from build123d import *

# Parameters (mm, degrees)
SKETCH_2_R          = 6
SKETCH_2_R_2        = 4
EXTRUDE_1_DEPTH     = 2
SKETCH_4_R          = 25
SKETCH_4_R_2        = 5
SKETCH_4_R_3        = 2
EXTRUDE_3_DEPTH     = 2
SKETCH_3_W          = 24
SKETCH_3_H          = 21.068287801
EXTRUDE_2_DEPTH     = 2
SKETCH_5_R          = 1.5
CUT_EXTRUDE_1_DEPTH = 50.779513859
FILLET_1_R          = 10


with BuildPart() as part:
    # 草图2 → 凸台-拉伸1 (new body)
    with BuildSketch(Plane(origin=(0, 0, 0), x_dir=(1, 0, 0), z_dir=(0, 1, 0))):
        with Locations(Location((0, 0, 0), (0, 0, 270))):
            Circle(SKETCH_2_R)
        with Locations(Location((0, 0, 0), (0, 0, 270))):
            Circle(SKETCH_2_R_2, mode=Mode.SUBTRACT)
    extrude(amount=EXTRUDE_1_DEPTH)

    # 草图4 → 凸台-拉伸3 (add)
    with BuildSketch(Plane(origin=(0, 2, 0), x_dir=(1, 0, 0), z_dir=(0, 1, 0))):
        with Locations(Location((0, 0, 0), (0, 0, 270))):
            Circle(SKETCH_4_R)
        Circle(SKETCH_4_R_2, mode=Mode.SUBTRACT)
        with Locations(Location((-10.253048327, 10.253048327, 0), (0, 0, 270))):
            Circle(SKETCH_4_R_3, mode=Mode.SUBTRACT)
        with Locations(Location((10.253048327, 10.253048327, 0), (0, 0, 270))):
            Circle(SKETCH_4_R_3, mode=Mode.SUBTRACT)
        with Locations(Location((-10.253048327, -10.253048327, 0), (0, 0, 270))):
            Circle(SKETCH_4_R_3, mode=Mode.SUBTRACT)
        with Locations(Location((10.253048327, -10.253048327, 0), (0, 0, 270))):
            Circle(SKETCH_4_R_3, mode=Mode.SUBTRACT)
    extrude(amount=-EXTRUDE_3_DEPTH)

    # 草图3 → 凸台-拉伸2 (add)
    with BuildSketch(Plane(origin=(0, 2, 0), x_dir=(1, 0, 0), z_dir=(0, 1, 0))):
        with Locations((0, -32.4658561)):
            Rectangle(SKETCH_3_W, SKETCH_3_H)
    extrude(amount=-EXTRUDE_2_DEPTH)

    # 草图5 → 切除-拉伸1 (cut, through all)
    with BuildSketch(Plane(origin=(0, 2, 0), x_dir=(1, 0, 0), z_dir=(0, 1, 0))):
        with Locations(Location((5, -28, 0), (0, 0, 270))):
            Circle(SKETCH_5_R)
        with Locations(Location((5, -38, 0), (0, 0, 270))):
            Circle(SKETCH_5_R)
        with Locations(Location((-5, -28, 0), (0, 0, 270))):
            Circle(SKETCH_5_R)
        with Locations(Location((-5, -38, 0), (0, 0, 270))):
            Circle(SKETCH_5_R)
    extrude(amount=-CUT_EXTRUDE_1_DEPTH, mode=Mode.SUBTRACT)

    # 圆角1
    fillet_1_edges = [part.edges().sort_by_distance(p)[0] for p in [
        (12, 1, 21.931712199),
        (-12, 1, 21.931712199),
    ]]
    fillet(fillet_1_edges, radius=FILLET_1_R)


solid = part.part
The model under review builds one solid part; all positions refer to its coordinate system, in mm. A direction names the side the tool comes from. Coordinates: 2 decimals unless noted, no trailing zeros. Loops run counter-clockwise (first coordinate to the right, second up) from the corner with the lowest first, then second, coordinate; pieces in that order, holes last. Notation, with made-up numbers: (11, 16.5) -> (48, 16.5) arc R13 cw to (48, 31.5) -> close; hole circle Ø2 at (-13.5, 64). An arc over 180 degrees is marked (long way). Use a Markdown table: item, result. Add a question column.
1. Add section C-C on z = 28. Write out the cut boundary in (x, y), plus the area to 3 significant figures.
2. Machinability: for faces 4 (the face through (12, 1, 35)), 5 (the face through (-12, 1, 35)), 6 (the face through (0, 0, 9)), which of the approach directions +Z, -Z, +X, -X, +Y, -Y give a long, thin tool a straight path to every point of the face, cutting with its end or side? Answer none if there is none.
3. To check wall thickness, follow line 1 (Z direction, x = 8.5, y = 0.1); line 2 (Z direction, x = -5.5, y = 1.5); line 3 (X direction, y = 0.3, z = 12). State the ranges of each line that lie inside material, in increasing order.
4. Add section A-A on z = 0. Write out the cut boundary in (x, y), plus the area to 3 significant figures.
5. Add section D-D on x = -5. Write out the cut boundary in (y, z), plus the area to 3 significant figures.
6. Draft analysis for pull direction X (two halves, no side actions). For faces 1 (the face through (13, 0.99, 22.86)), 2 (the face through (5.07, 1.01, 26.5)), 3 (the face through (0.861, 1.014, -24.985)), state which applies: pulls with the +X half, pulls with the -X half, needs draft (parallel to the pull), parting line crosses it, or undercut.
7. Add section B-B on x = 0. Write out the cut boundary in (y, z).
Returned:
| question | item | result |
|---|---|---|
| 1 | outline | (-12, 0) -> (-6.5, 0) -> (-6.5, 2) -> (-12, 2) -> close; (-3.5, 0) -> (3.5, 0) -> (3.5, 2) -> (-3.5, 2) -> close; (6.5, 0) -> (12, 0) -> (12, 2) -> (6.5, 2) -> close |
| 1 | area | 36.0 mm² |
| 2 | face 4 | +Z, +X, +Y, -Y |
| 2 | face 5 | +Z, -X, +Y, -Y |
| 2 | face 6 | +Z, -Z, +X, -X, -Y |
| 3 | line 1 | z = -23.51 to -11.22, -9.29 to 9.29, 11.22 to 43 |
| 3 | line 2 | z = -24.39 to 26.59, 29.41 to 36.59, 39.41 to 43 |
| 3 | line 3 | x = -21.93 to -11.23, -9.28 to 9.28, 11.23 to 21.93 |
| 4 | outline | (-25, 0) -> (-4, 0) -> (-4, 2) -> (-25, 2) -> close; (4, 0) -> (25, 0) -> (25, 2) -> (4, 2) -> close |
| 4 | area | 84.0 mm² |
| 5 | outline | (0, -24.49) -> (2, -24.49) -> (2, 26.5) -> (0, 26.5) -> close; (0, 29.5) -> (2, 29.5) -> (2, 36.5) -> (0, 36.5) -> close; (0, 39.5) -> (2, 39.5) -> (2, 43) -> (0, 43) -> close |
| 5 | area | 123 mm² |
| 6 | face 1 | pulls with the +X half |
| 6 | face 2 | undercut |
| 6 | face 3 | parting line crosses it |
| 7 | outline | (0, -25) -> (2, -25) -> (2, -4) -> (0, -4) -> close; (0, 4) -> (2, 4) -> (2, 43) -> (0, 43) -> close |
